CAD build for the part. Positions are in the model's coordinates, mm. Face numbers are marked on the shaded views. A direction names the side the tool comes from. Give positions to 0.01 mm unless a question says otherwise; leave off trailing zeros. Write each loop counter-clockwise with the first axis right and the second up, starting at its lowest first coordinate (ties: lowest second). Pieces come first, ordered by that corner, then holes. Notation, with made-up numbers: (58.25, 62.5) - (95.25, 62.5) arc R25 ccw to (95.25, 91.5) - close; hole circle Ø5 at (-33, -5). An arc over 180 degrees is marked (long way). Put each result on its own line as item: value. Start each with the question number.
1. Cut at A-A on z = 16. List the corners of the cut face in (x, y), and give its area (3 significant figures).
2. Wall check: line 1 (X direction, y = -3, z = -32); line 2 (X direction, y = 79, z = -29); line 3 (Z direction, x = 23.5, y = 81). Give the ranges that are in metal, low to high.
3. Cut at C-C on y = 87. List the corners of the cut face in (x, z), and give its area (3 significant figures).
4. Cut at D-D on x = 29. List the corners of the cut face in (y, z).
5. Drop flat-ended pins along their axis: pin 1 (4 mm diameter, centred on x = -52, y = -7.5, fed in from -Z); pin 2 (4 mm diameter, centred on x = 51, z = -16.5, fed in from -Y); pin 3 (2 mm diameter, centred on x = -43, y = 3.5, fed in from +Z). Give the stop position or say it passes through.
6. Tool access for the marked faces 1, 2 and 3: list every direction of +Z, -Z, +X, -X, +Y, -Y with a clear straight run to the whole face (end or side of a thin tool).
7. Cut at B-B on y = 0.5. List the corners of the cut face in (x, z), and give its area (3 significant figures).
from build123d import *

# Parameters (mm, degrees)
F0_W     = 24.9655246735
F0_H     = 18.6489485204
F1_DEPTH = 25.4
F2_W     = 24.9655246735
F2_H     = 18.6489485204
F3_DEPTH = 69.088
F4_W     = 24.9655246735
F4_H     = 18.6489485204
F5_DEPTH = 7.62
F4_W_2   = 13.3254788816
F4_H_2   = 182.7494688332
F6_DEPTH = 10.922
F7_DEPTH = 131.318


with BuildPart() as f1:
    # F0 (on Top) → F1 (new body)
    with BuildSketch(Plane.XY):
        with Locations((0.7519731298, 1.203157939)):
            Rectangle(F0_W, F0_H)
    extrude(amount=F1_DEPTH)

    # F2 (on face) → F3 (join)
    with BuildSketch(Plane(origin=(0, 0, 0), x_dir=(1, 0, 0), z_dir=(0, 0, -1))):
        with Locations((0.7519731298, -1.203157939)):
            Rectangle(F2_W, F2_H)
    extrude(amount=F3_DEPTH)

    # F4 (on face) → F5 (join)
    with BuildSketch(Plane(origin=(0, 0, -69.088), x_dir=(1, 0, 0), z_dir=(0, 0, -1))):
        Polygon((46.6391891241, 47.2034774721), (-78.5251632333, 47.2034774721), (-78.5251632333, -136.0218971968), (46.6391891241, -136.0218971968), (46.6391891241, 46.7275716364), align=None)
        with Locations((0.7519731298, -1.203157939)):
            Rectangle(F4_W, F4_H, mode=Mode.SUBTRACT)
        with Locations((0.7519731298, -1.203157939)):
            Rectangle(F4_W, F4_H)
    extrude(amount=F5_DEPTH)

    # F4 (on face) → F6 (join, symmetric)
    with BuildSketch(Plane(origin=(0, 0, -69.088), x_dir=(1, 0, 0), z_dir=(0, 0, -1))):
        with Locations((53.3019285649, -44.6471627802)):
            Rectangle(F4_W_2, F4_H_2)
    extrude(amount=F6_DEPTH, both=True)

    # F7 (add): a face of the model
    f7_faces = [f1.faces().sort_by_distance(p)[0] for p in [
        (53.3019285649, 44.6471627802, -58.166),
    ]]
    extrude(f7_faces, amount=F7_DEPTH)


solid = f1.part
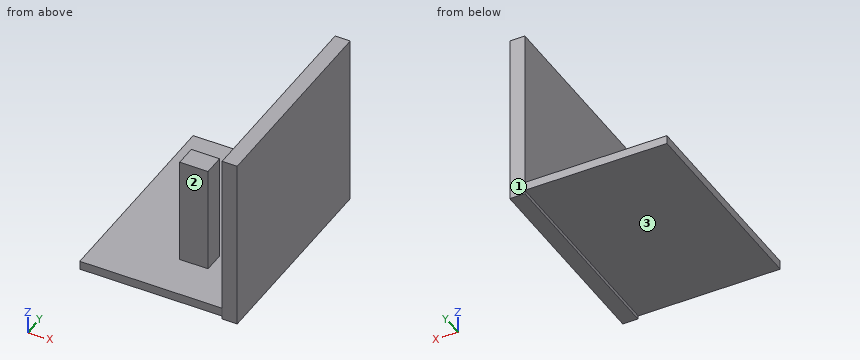
Report:
1. outline: (-11.73, -8.12) - (13.23, -8.12) - (13.23, 10.53) - (-11.73, 10.53) - close; (46.64, -46.73) - (59.96, -46.73) - (59.96, 136.02) - (46.64, 136.02) - close
1. area: 2,900 mm²
2. line 1: x = -11.73 to 13.23, 46.64 to 59.96
2. line 2: x = 46.64 to 59.96
2. line 3: z = -76.71 to -69.09
3. outline: (-78.53, -76.71) - (46.64, -76.71) - (46.64, -80.01) - (59.96, -80.01) - (59.96, 73.15) - (46.64, 73.15) - (46.64, -69.09) - (-78.53, -69.09) - close
3. area: 2,990 mm²
4. outline: (-47.2, -76.71) - (136.02, -76.71) - (136.02, -69.09) - (-47.2, -69.09) - close
5. pin 1: stops at z = -76.71
5. pin 2: stops at y = -46.73
5. pin 3: stops at z = -69.09
6. face 1: +Z, -Z, +X, -X, +Y
6. face 2: +Z, -X, -Y
6. face 3: -Z, -X, +Y, -Y
7. outline: (-78.53, -76.71) - (46.64, -76.71) - (46.64, -80.01) - (59.96, -80.01) - (59.96, 73.15) - (46.64, 73.15) - (46.64, -69.09) - (13.23, -69.09) - (13.23, 25.4) - (-11.73, 25.4) - (-11.73, -69.09) - (-78.53, -69.09) - close
7. area: 5,350 mm²
